Part model, mm, in its own coordinate system. A direction names the side the tool comes from. Give positions to 0.01 mm unless a question says otherwise; leave off trailing zeros. Write each loop counter-clockwise with the first axis right and the second up, starting at its lowest first coordinate (ties: lowest second). Pieces come first, ordered by that corner, then holes.
from build123d import *
from build123d.topology import SkipClean

# Parameters (mm, degrees)
SALIENTE_EXTRUIR1_DEPTH      = 106
SALIENTE_EXTRUIR2_DEPTH      = 5
SALIENTE_EXTRUIR2_DEPTH_BACK = 110
CROQUIS2_R                   = 77.5
SALIENTE_EXTRUIR3_DEPTH      = 52.5
SALIENTE_EXTRUIR3_DEPTH_BACK = 126
CROQUIS3_R                   = 55


with BuildPart() as part:
    # Croquis1 → Saliente-Extruir1 (new body)
    with BuildSketch(Plane(origin=(0, 0, 0), x_dir=(1, 0, 0), z_dir=(0, 1, 0))):
        with BuildLine():
            Line((62.371868659, 46), (372.350129794, 46))
            ThreePointArc((372.350129794, 46), (457.499756657, 0), (372.350129794, -46))
            Line((372.350129794, -46), (62.371868659, -46))
            ThreePointArc((62.371868659, -46), (-77.5, 0), (62.371868659, 46))
        make_face()
    extrude(amount=SALIENTE_EXTRUIR1_DEPTH)

    # Croquis2 → Saliente-Extruir2 (add, two sides: drawn at the far end of the back side and taken through both)
    with SkipClean():  # the faces are left unmerged after this step: merging them gives an invalid solid
        with BuildSketch(Plane(origin=(0, 106, 0), x_dir=(1, 0, 0), z_dir=(0, 1, 0)).offset(-SALIENTE_EXTRUIR2_DEPTH_BACK)):
            with Locations(Location((0, 0, 0), (0, 0, 270))):
                Circle(CROQUIS2_R)
        extrude(amount=SALIENTE_EXTRUIR2_DEPTH + SALIENTE_EXTRUIR2_DEPTH_BACK)
    add(part.part.scale(1), mode=Mode.REPLACE)  # the faces are merged on a copy

    # Croquis3 → Saliente-Extruir3 (add, two sides: drawn at the far end of the back side and taken through both)
    with SkipClean():  # the faces are left unmerged after this step: merging them gives an invalid solid
        with BuildSketch(Plane(origin=(0, 106, 0), x_dir=(1, 0, 0), z_dir=(0, 1, 0)).offset(-SALIENTE_EXTRUIR3_DEPTH_BACK)):
            with Locations(Location((402.499756657, 0, 0), (0, 0, 270))):
                Circle(CROQUIS3_R)
        extrude(amount=SALIENTE_EXTRUIR3_DEPTH + SALIENTE_EXTRUIR3_DEPTH_BACK)
    add(part.part.scale(1), mode=Mode.REPLACE)  # the faces are merged on a copy


solid = part.part
1) Mould opens along X. For faces 1 (the flat face through (1, 111, -1)), 2 (the flat face through (220, 106, -1)) say: +X half, -X half, draft (parallel to the pull), parting line (faces both ways), or undercut.
Check result:
face 1: draft
face 2: undercut
2) Saw through at A-A (z = 0). Write the cut outline in (x, y), and give its area (3 significant figures).
Check result:
outline: (-77.5, -4) - (77.5, -4) - (77.5, 0) - (347.5, 0) - (347.5, -20) - (457.5, -20) - (457.5, 158.5) - (347.5, 158.5) - (347.5, 106) - (77.5, 106) - (77.5, 111) - (-77.5, 111) - close
area: 66,100 mm2
3) Flat gauge pins, fed straight in: P1, Ø2, axis at y = 22.5, z = 7, coming from the -X side; P2, Ø1, axis at x = 389, y = 3.5, coming from the +Z side; P3, Ø6, axis at x = 57, y = 93, coming from the -Z side. Where does each tip first touch, or does it go through?
Check result:
P1: stops at x = -77.27
P2: stops at z = 53.44
P3: stops at z = -55.59
4) Drill centre lines: L1, parallel to Y at x = 224, z = -4; L2, parallel to Z at x = 108, y = 22; L3, parallel to Z at x = -1, y = 101.5. Where is each one in solid material? Low to high.
Check result:
L1: y = 0 to 106
L2: z = -46 to 46
L3: z = -77.49 to 77.49
5) Saw through at D-D (y = 120). Write the cut outline in (x, z), and give its area (3 significant figures).
Check result:
outline: circle Ø110 at (402.5, 0)
area: 9,500 mm2
6) Saw through at B-B (x = 71.5). Write the cut outline in (y, z).
Check result:
outline: (-4, -29.9) - (0, -29.9) - (0, -46) - (106, -46) - (106, -29.9) - (111, -29.9) - (111, 29.9) - (106, 29.9) - (106, 46) - (0, 46) - (0, 29.9) - (-4, 29.9) - close
7) Saw through at C-C (y = 84). Write the cut outline in (x, z).
Check result:
outline: (62.37, -46) - (372.35, -46) arc R55 ccw (long way) to (372.35, 46) - (62.37, 46) arc R77.5 ccw (long way) to start
8) 3-axis set-ups, long thin cutter, end or side, ignore diameter. For faces 3 (the flat face through (403, 158.5, -1)), 4 (the flat face through (220, 52, 46)), 5 (the flat face through (1, -4, -1)), 6 (the flat face through (215, 52, -46)): which of +Z, -Z, +X, -X, +Y, -Y reach the whole face in a straight line?
Check result:
face 3: +Z, -Z, +X, -X, +Y
face 4: +Z, +Y, -Y
face 5: +Z, -Z, -X, -Y
face 6: -Z, +Y, -Y
